The model under review builds one solid part; all positions refer to its coordinate system, in mm. Face numbers are marked on the shaded views. Round coordinates to 2 decimals unless told otherwise and drop trailing zeros. Write each loop counter-clockwise with the first axis right and the second up, starting at its lowest first coordinate (ties: lowest second). Pieces come first, ordered by that corner, then holes. Notation, with made-up numbers: (13.25, 55) -> (42.25, 55) arc R26 cw to (42.25, 71) -> close; hole circle Ø7 at (-19.75, -37.5). An arc over 180 degrees is marked (long way). Return JSON: item names as keys, results as strings. Group by question number.
1. Take a section at B-B, the plane z = 0. Give the number of separate pieces and of enclosed holes in the cut face, then the cut area to 3 significant figures.
2. Clearance check with flat-ended pins moving along their axes: P1, Ø4, axis at x = 208, z = -2.5, coming from the -Y side; P2, Ø8, axis at x = 115.5, y = 6, coming from the -Z side; P3, Ø4.5, axis at x = -5, z = -0.5, coming from the -Y side; P4, Ø3, axis at x = 56.5, y = -11.5, coming from the -Z side. State where each tip first meets the part, or that it passes through.
3. For line 1 along X through (y, z) = (11, -0.5); line 2 along Y through (x, z) = (137.5, 0.75); line 3 along Z through (x, y) = (149.5, -0.5), list the stretches that pass through material, from the lowest coordinate up. Write a range as from..to.
4. Take a section at A-A, the plane y = 0. Write out the cut boundary in (x, z), then the cut area to 3 significant figures.
5. Mouldability with a two-part tool opening along Z and no side actions: class the marked faces 1 and 2 as pulls with the +Z half, pulls with the -Z half, needs draft (parallel to the pull), parting line crosses it, or undercut.
6. Take a section at C-C, the plane x = 13. Write out the cut boundary in (y, z), then the cut area to 3 significant figures.
from build123d import *

# Parameters (mm, degrees)
ESBO_O1_R                  = 15
ESBO_O1_R_2                = 12.5
RESSALTO_EXTRUS_O1_DEPTH   = 210
RESSALTO_EXTRUS_O3_START   = 10
ESBO_O2_R                  = 12.5
ESBO_O2_R_2                = 10
RESSALTO_EXTRUS_O3_DEPTH   = 15
CORTE_EXTRUS_O3_DEPTH      = 300
CORTE_EXTRUS_O3_DEPTH_BACK = 300
ESBO_O4_R                  = 2.5
RESSALTO_EXTRUS_O4_START   = -5
ESBO_O9_R                  = 12.5
RESSALTO_EXTRUS_O4_DEPTH   = 5
FILETE1_R                  = 1
ESBO_O11_W                 = 15
ESBO_O11_H                 = 10
CORTE_EXTRUS_O4_DEPTH      = 10


with BuildPart() as part:
    # Esbo_o1 → Ressalto-extrus_o1 (new body)
    with BuildSketch(Plane(origin=(0, 0, 0), x_dir=(0, 0, -1), z_dir=(1, 0, 0))):
        Circle(ESBO_O1_R)
        Circle(ESBO_O1_R_2, mode=Mode.SUBTRACT)
    extrude(amount=RESSALTO_EXTRUS_O1_DEPTH)

    # Esbo_o2 → Ressalto-extrus_o3 (add)
    with BuildSketch(Plane.ZY.offset(RESSALTO_EXTRUS_O3_START)):
        Circle(ESBO_O2_R)
        Circle(ESBO_O2_R_2, mode=Mode.SUBTRACT)
    extrude(amount=-RESSALTO_EXTRUS_O3_DEPTH)

    # Esbo_o4 → Corte-extrus_o3 (cut, two sides: drawn at the far end of the back side and taken through both)
    with BuildSketch(Plane(origin=(0, 0, 0), x_dir=(1, 0, 0), z_dir=(0, 1, 0)).offset(-CORTE_EXTRUS_O3_DEPTH_BACK)):
        with Locations(Location((-5, 0.5, 0), (0, 0, 90))):
            Circle(ESBO_O4_R)
    extrude(amount=CORTE_EXTRUS_O3_DEPTH + CORTE_EXTRUS_O3_DEPTH_BACK, mode=Mode.SUBTRACT)

    # Esbo_o9 → Ressalto-extrus_o4 (add)
    with BuildSketch(Plane(origin=(210, 0, 0), x_dir=(0, 0, -1), z_dir=(1, 0, 0)).offset(RESSALTO_EXTRUS_O4_START)):
        with Locations(Location((0, 0, 0), (0, 0, 180))):
            Circle(ESBO_O9_R)
    extrude(amount=RESSALTO_EXTRUS_O4_DEPTH)

    # Filete1
    filete1_edges = [part.edges().sort_by_distance(p)[0] for p in [
        (210, 0, 15),
    ]]
    fillet(filete1_edges, radius=FILETE1_R)

    # Esbo_o11 → Corte-extrus_o4 (cut)
    with BuildSketch(Plane(origin=(210, 0, 0), x_dir=(0, 0, -1), z_dir=(1, 0, 0))):
        Rectangle(ESBO_O11_W, ESBO_O11_H)
    extrude(amount=-CORTE_EXTRUS_O4_DEPTH, mode=Mode.SUBTRACT)


solid = part.part
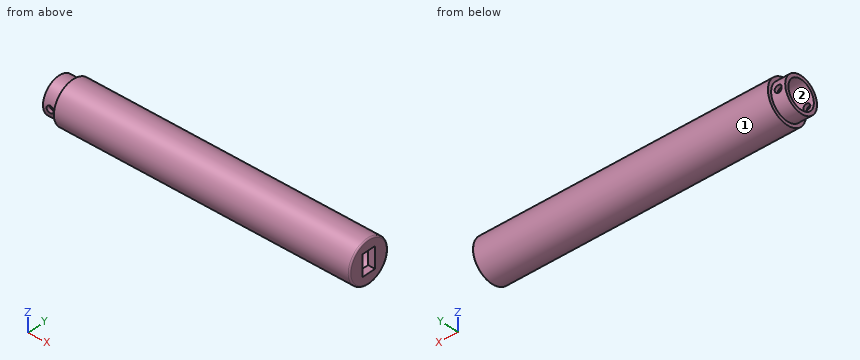
Output:
{
 "1": {"separate pieces": "4", "enclosed holes": "0", "area": "1,180 mm^2"},
 "2": {"P1": "stops at y = -14.99", "P2": "stops at z = -14.87", "P3": "passes through", "P4": "stops at z = -11.18"},
 "3": {"line 1": "x = -10..-7.5, -2.5..5, 205..210", "line 2": "y = -14.98..-12.48, 12.48..14.98", "line 3": "z = -14.99..-12.49, 12.49..14.99"},
 "4": {"outline": "(-10, -12.5) -> (0, -12.5) -> (0, -15) -> (209, -15) arc R1 ccw to (210, -14) -> (210, -7.5) -> (205, -7.5) -> (205, -12.5) -> (5, -12.5) -> (5, -10) -> (-10, -10) -> close; (-10, 10) -> (5, 10) -> (5, 12.5) -> (205, 12.5) -> (205, 7.5) -> (210, 7.5) -> (210, 14) arc R1 ccw to (209, 15) -> (0, 15) -> (0, 12.5) -> (-10, 12.5) -> close", "area": "1,170 mm^2"},
 "5": {"face 1": "parting line crosses it", "face 2": "undercut"},
 "6": {"outline": "circle Ø30 at (0, 0); hole circle Ø25 at (0, 0)", "area": "216 mm^2"}
}
